Design review of the part built by this model. Coordinates are the model's own, in mm. A direction names the side the tool comes from. Give positions to 0.01 mm unless a question says otherwise; leave off trailing zeros. Loops run counter-clockwise (first coordinate to the right, second up) from the corner with the lowest first, then second, coordinate; pieces in that order, holes last. Notation, with made-up numbers: (-10, 49.25) -> (20, 49.25) arc R22 ccw to (20, 85.25) -> close; hole circle Ø8 at (7.25, -30). An arc over 180 degrees is marked (long way). Use CSV: the item, a comma, the result in double quotes. Start each with the question number.
Item 1: We need section A-A (z = 8.75). State the section outline as (x, y) points.
Item 2: Clearance check with flat-ended pins moving along their axes: pin 1 (4 mm diameter, centred on x = 1.5, z = -1.5, fed in from -Y); pin 2 (2 mm diameter, centred on x = 3, y = -5, fed in from -Z); pin 3 (2 mm diameter, centred on x = 0, z = -8.75, fed in from -Y); pin 4 (2.5 mm diameter, centred on x = 0.5, z = -0.5, fed in from -Y). State where each tip first meets the part, or that it passes through.
Item 3: The part is to be moulded in two halves that separate along X. For faces 1 (the face through (-3.046, 0.507, -8.311)), 2 (the face through (3, -10, 0)), 3 (the face through (-0.098, 0.507, -13.494)), say which applies: +X half, -X half, draft (parallel to the pull), parting line (faces both ways), or undercut.
Item 4: Wall thickness on line 1 along Z through (x, y) = (-3, -6); line 2 along Y through (x, z) = (-1.25, 0); line 3 along Z through (x, y) = (0.5, -3.25): over which ranges is each line inside the solid? List them lowest first. Write a range as from..to.
Item 5: We need section C-C (y = -5.75). State the section outline as (x, z) points, plus the area to 3 significant figures.
Item 6: We need section B-B (x = 3). State the section outline as (y, z) points, plus the area to 3 significant figures.
Item 7: For faces 4 (the face through (1, 0.5, -1)), 5 (the face through (-3.68, 0.51, -0.02)), 6 (the face through (3.68, 0.51, 0.02)), list the 3-axis set-ups (+Z, -Z, +X, -X, +Y, -Y) from which the entire face can be reached by the end or side of a thin tool; tool diameter is ignored.
Item 8: We need section D-D (z = -10.75). State the section outline as (x, y) points.
from build123d import *

# Parameters (mm, degrees)
BOSS_EXTRUDE1_DEPTH             = 1
SKETCH2_R                       = 3.75
BOSS_EXTRUDE2_DEPTH             = 10
CUT_EXTRUDE1_DEPTH              = 3
DRAFT1_ANGLE                    = 6.428571429
DRAFT2_ANGLE                    = 6.428571429
DRAFT3_ANGLE                    = 6.428571429
DRAFT4_ANGLE                    = 6.428571429
DRAFT5_ANGLE                    = 6.428571429
DRAFT6_ANGLE                    = 6.428571429
DRAFT7_ANGLE                    = 6.428571429
DRAFT8_ANGLE                    = 6.428571429
F_1_5_1_5_DIAMETER_HOLE1_D      = 1.5
M5X0_8_TAPPED_HOLE1_D           = 1.5
M5X0_8_TAPPED_HOLE1_DEPTH       = 11
M5X0_8_TAPPED_HOLE1_CBORE_D     = 5
M5X0_8_TAPPED_HOLE1_CBORE_DEPTH = 0.5


with BuildPart() as part:
    # Sketch1 → Boss-Extrude1 (new body)
    with BuildSketch(Plane(origin=(0, 1, 0), x_dir=(1, 0, 0), z_dir=(0, 1, 0))):
        with BuildLine():
            Line((-2.5, 14.75), (-3.606876141, 1.688861534))
            ThreePointArc((-3.606876141, 1.688861534), (-3.678310043, 0), (-3.606876141, -1.688861534))
            Line((-3.606876141, -1.688861534), (-2.5, -14.75))
            ThreePointArc((-2.5, -14.75), (0, -17.25), (2.5, -14.75))
            Line((2.5, -14.75), (3.606876141, -1.688861534))
            ThreePointArc((3.606876141, -1.688861534), (3.678310043, 0), (3.606876141, 1.688861534))
            Line((3.606876141, 1.688861534), (2.5, 14.75))
            ThreePointArc((2.5, 14.75), (0, 17.25), (-2.5, 14.75))
        make_face()
    extrude(amount=-BOSS_EXTRUDE1_DEPTH)

    # Sketch2 → Boss-Extrude2 (add)
    with BuildSketch(Plane.XZ):
        with Locations(Location((0, 0, 0), (0, 0, 12.437280395))):
            Circle(SKETCH2_R)
    extrude(amount=BOSS_EXTRUDE2_DEPTH)

    # Sketch3 → Cut-Extrude1 (cut)
    with BuildSketch(Plane.XZ.offset(10)):
        Polygon((0.132515428, 2.359655809), (0, 2.492171237), (-0.132515428, 2.359655809), (-0.279034647, 2.476500987), (-0.395879825, 2.329981768), (-0.554560271, 2.4296873), (-0.654265804, 2.271006854), (-0.823111978, 2.352318886), (-0.90442401, 2.183472712), (-1.081312575, 2.245368698), (-1.14320856, 2.068480133), (-1.325915038, 2.110181695), (-1.367616599, 1.927475217), (-1.574826066, 1.950822117), (-1.574826066, 1.762231181), (-1.762231181, 1.762231181), (-1.762231181, 1.574826066), (-1.950822117, 1.574826066), (-1.927475217, 1.367616599), (-2.110181695, 1.325915038), (-2.068480133, 1.14320856), (-2.245368698, 1.081312575), (-2.183472712, 0.90442401), (-2.352318886, 0.823111978), (-2.271006854, 0.654265804), (-2.4296873, 0.554560271), (-2.329981768, 0.395879825), (-2.476500987, 0.279034647), (-2.359655809, 0.132515428), (-2.492171237, 0), (-2.359655809, -0.132515428), (-2.476500987, -0.279034647), (-2.329981768, -0.395879825), (-2.4296873, -0.554560271), (-2.271006854, -0.654265804), (-2.352318886, -0.823111978), (-2.183472712, -0.90442401), (-2.245368698, -1.081312575), (-2.068480133, -1.14320856), (-2.110181695, -1.325915038), (-1.927475217, -1.367616599), (-1.950822117, -1.574826066), (-1.762231181, -1.574826066), (-1.762231181, -1.762231181), (-1.574826066, -1.762231181), (-1.574826066, -1.950822117), (-1.367616599, -1.927475217), (-1.325915038, -2.110181695), (-1.14320856, -2.068480133), (-1.081312575, -2.245368698), (-0.90442401, -2.183472712), (-0.823111978, -2.352318886), (-0.654265804, -2.271006854), (-0.554560271, -2.4296873), (-0.395879825, -2.329981768), (-0.279034647, -2.476500987), (-0.132515428, -2.359655809), (0, -2.492171237), (0.132515428, -2.359655809), (0.279034647, -2.476500987), (0.395879825, -2.329981768), (0.554560271, -2.4296873), (0.654265804, -2.271006854), (0.823111978, -2.352318886), (0.90442401, -2.183472712), (1.081312575, -2.245368698), (1.14320856, -2.068480133), (1.325915038, -2.110181695), (1.367616599, -1.927475217), (1.574826066, -1.950822117), (1.574826066, -1.762231181), (1.762231181, -1.762231181), (1.762231181, -1.574826066), (1.950822117, -1.574826066), (1.927475217, -1.367616599), (2.110181695, -1.325915038), (2.068480133, -1.14320856), (2.245368698, -1.081312575), (2.183472712, -0.90442401), (2.352318886, -0.823111978), (2.271006854, -0.654265804), (2.4296873, -0.554560271), (2.329981768, -0.395879825), (2.476500987, -0.279034647), (2.359655809, -0.132515428), (2.492171237, 0), (2.359655809, 0.132515428), (2.476500987, 0.279034647), (2.329981768, 0.395879825), (2.4296873, 0.554560271), (2.271006854, 0.654265804), (2.352318886, 0.823111978), (2.183472712, 0.90442401), (2.245368698, 1.081312575), (2.068480133, 1.14320856), (2.110181695, 1.325915038), (1.927475217, 1.367616599), (1.950822117, 1.574826066), (1.762231181, 1.574826066), (1.762231181, 1.762231181), (1.574826066, 1.762231181), (1.574826066, 1.950822117), (1.367616599, 1.927475217), (1.325915038, 2.110181695), (1.14320856, 2.068480133), (1.081312575, 2.245368698), (0.90442401, 2.183472712), (0.823111978, 2.352318886), (0.654265804, 2.271006854), (0.554560271, 2.4296873), (0.395879825, 2.329981768), (0.279034647, 2.476500987), align=None)
    extrude(amount=-CUT_EXTRUDE1_DEPTH, mode=Mode.SUBTRACT)

    # Draft1
    draft1_faces = [part.faces().sort_by_distance(p)[0] for p in [
        (1.856526649, -8.5, 1.574826066),
    ]]
    draft(draft1_faces, Plane(origin=(1.762231181, -7, 1.574826066), x_dir=(0, 0, -1), z_dir=(-1, 0, 0)), DRAFT1_ANGLE)

    # Draft2
    draft2_faces = [part.faces().sort_by_distance(p)[0] for p in [
        (1.574826066, -8.5, 1.856526649),
    ]]
    draft(draft2_faces, Plane(origin=(1.762231181, -7, 1.762231181), x_dir=(-1, 0, 0), z_dir=(0, 0, -1)), DRAFT2_ANGLE)

    # Draft3
    draft3_faces = [part.faces().sort_by_distance(p)[0] for p in [
        (1.574826066, -8.5, -1.856526649),
    ]]
    draft(draft3_faces, Plane(origin=(1.574826066, -7, -1.762231181), x_dir=(1, 0, 0), z_dir=(0, 0, 1)), DRAFT3_ANGLE)

    # Draft4
    draft4_faces = [part.faces().sort_by_distance(p)[0] for p in [
        (1.856526649, -8.5, -1.574826066),
    ]]
    draft(draft4_faces, Plane(origin=(1.762231181, -7, -1.762231181), x_dir=(0, 0, -1), z_dir=(-1, 0, 0)), DRAFT4_ANGLE)

    # Draft5
    draft5_faces = [part.faces().sort_by_distance(p)[0] for p in [
        (-1.856526649, -8.5, -1.574826066),
    ]]
    draft(draft5_faces, Plane(origin=(-1.762231181, -7, -1.574826066), x_dir=(0, 0, 1), z_dir=(1, 0, 0)), DRAFT5_ANGLE)

    # Draft6
    draft6_faces = [part.faces().sort_by_distance(p)[0] for p in [
        (-1.574826066, -8.5, -1.856526649),
    ]]
    draft(draft6_faces, Plane(origin=(-1.762231181, -7, -1.762231181), x_dir=(1, 0, 0), z_dir=(0, 0, 1)), DRAFT6_ANGLE)

    # Draft7
    draft7_faces = [part.faces().sort_by_distance(p)[0] for p in [
        (-1.574826066, -8.5, 1.856526649),
    ]]
    draft(draft7_faces, Plane(origin=(-1.574826066, -7, 1.762231181), x_dir=(-1, 0, 0), z_dir=(0, 0, -1)), DRAFT7_ANGLE)

    # Draft8
    draft8_faces = [part.faces().sort_by_distance(p)[0] for p in [
        (-1.856526649, -8.5, 1.574826066),
    ]]
    draft(draft8_faces, Plane(origin=(-1.762231181, -7, 1.762231181), x_dir=(0, 0, 1), z_dir=(1, 0, 0)), DRAFT8_ANGLE)

    # Ø1.5 (1.5) Diameter Hole1 (through all)
    with Locations(Plane(origin=(0, 0, 0), x_dir=(-1, 0, 0), z_dir=(0, -1, 0))):
        with Locations((0, 14.75), (0, 12.75), (0, 10.75), (0, 8.75), (0, 6.75), (0, 4.75), (0, -4.75), (0, -6.75), (0, -8.75), (0, -10.75), (0, -12.75), (0, -14.75)):
            Hole(F_1_5_1_5_DIAMETER_HOLE1_D / 2)

    # M5x0.8 Tapped Hole1
    with Locations(Plane(origin=(0, 1, 0), x_dir=(1, 0, 0), z_dir=(0, 1, 0))):
        with Locations((0, 0)):
            CounterBoreHole(M5X0_8_TAPPED_HOLE1_D / 2, M5X0_8_TAPPED_HOLE1_CBORE_D / 2, M5X0_8_TAPPED_HOLE1_CBORE_DEPTH, depth=M5X0_8_TAPPED_HOLE1_DEPTH)


solid = part.part
Results found:
1,outline,"(-3.01, 0) -> (-0.75, 0) -> (-0.75, 1) -> (-3.01, 1) -> close; (0.75, 0) -> (3.01, 0) -> (3.01, 1) -> (0.75, 1) -> close"
2,pin 1,"y = -10"
2,pin 2,"z = -3.17"
2,pin 3,"y = 0"
2,pin 4,"y = -7"
3,face 1,"-X half"
3,face 2,"draft"
3,face 3,"undercut"
4,line 1,"-2.25..2.25"
4,line 2,"-7..0.5"
4,line 3,"-3.72..-0.56, 0.56..3.72"
5,outline,"circle Ø7.5 at (0, 0); hole circle Ø1.5 at (0, 0)"
5,area,"42.4 mm²"
6,outline,"(-10, -2.25) -> (0, -2.25) -> (0, -8.85) -> (1, -8.85) -> (1, 8.85) -> (0, 8.85) -> (0, 2.25) -> (-10, 2.25) -> close"
6,area,"62.7 mm²"
7,face 4,"+Y"
7,face 5,"-X, +Y"
7,face 6,"+X, +Y"
8,outline,"(-2.84, 0) -> (-0.75, 0) -> (-0.75, 1) -> (-2.84, 1) -> close; (0.75, 0) -> (2.84, 0) -> (2.84, 1) -> (0.75, 1) -> close"
